Design review of the part built by this model. Coordinates are the model's own, in mm. Face numbers are marked on the shaded views. A direction names the side the tool comes from. Coordinates: 2 decimals unless noted, no trailing zeros. Loops run counter-clockwise (first coordinate to the right, second up) from the corner with the lowest first, then second, coordinate; pieces in that order, holes last. Notation, with made-up numbers: (-39.5, 29) -> (8.5, 29) arc R14 cw to (8.5, 35) -> close; hole circle Ø7 at (71, 21). An arc over 180 degrees is marked (long way). Answer in a Markdown table with one row per item.
```python
from build123d import *

# Parameters (mm, degrees)
SKETCH_1_R      = 9.9
SKETCH_1_R_2    = 1.85
EXTRUDE_1_DEPTH = 7
SKETCH_2_R      = 12.5
SKETCH_2_R_2    = 1.85
EXTRUDE_2_DEPTH = 2.5
SKETCH_3_R      = 3.75
EXTRUDE_3_DEPTH = 6.3
CHAMFER_1_SIZE  = 2


with BuildPart() as part:
    # 草图1 → 凸台-拉伸1 (new body)
    with BuildSketch(Plane(origin=(0, 0, 0), x_dir=(1, 0, 0), z_dir=(0, 1, 0))):
        with Locations(Location((0, 0, 0), (0, 0, 270))):
            Circle(SKETCH_1_R)
        with Locations(Location((6, 0, 0), (0, 0, 270))):
            Circle(SKETCH_1_R_2, mode=Mode.SUBTRACT)
        with Locations(Location((0, -6, 0), (0, 0, 270))):
            Circle(SKETCH_1_R_2, mode=Mode.SUBTRACT)
        with Locations(Location((-6, 0, 0), (0, 0, 270))):
            Circle(SKETCH_1_R_2, mode=Mode.SUBTRACT)
        with Locations(Location((0, 6, 0), (0, 0, 270))):
            Circle(SKETCH_1_R_2, mode=Mode.SUBTRACT)
    extrude(amount=EXTRUDE_1_DEPTH)

    # 草图2 → 凸台-拉伸2 (add)
    with BuildSketch(Plane(origin=(0, 7, 0), x_dir=(1, 0, 0), z_dir=(0, 1, 0))):
        with Locations(Location((0, 0, 0), (0, 0, 270))):
            Circle(SKETCH_2_R)
        with Locations(Location((-6, 0, 0), (0, 0, 270))):
            Circle(SKETCH_2_R_2, mode=Mode.SUBTRACT)
        with Locations(Location((0, -6, 0), (0, 0, 270))):
            Circle(SKETCH_2_R_2, mode=Mode.SUBTRACT)
        with Locations(Location((6, 0, 0), (0, 0, 270))):
            Circle(SKETCH_2_R_2, mode=Mode.SUBTRACT)
        with Locations(Location((0, 6, 0), (0, 0, 270))):
            Circle(SKETCH_2_R_2, mode=Mode.SUBTRACT)
    extrude(amount=EXTRUDE_2_DEPTH)

    # 草图3 → 凸台-拉伸3 (add)
    # profile 1 of 8: a face of its own
    with BuildSketch(Plane(origin=(0, 9.5, 0), x_dir=(1, 0, 0), z_dir=(0, 1, 0))):
        with BuildLine():
            Line((2.25, 0), (-2.25, 0))
            ThreePointArc((-2.25, 0), (-6, -3.75), (-9.75, 0))
            Line((-9.75, 0), (-12.5, 0))
            ThreePointArc((-12.5, 0), (-3.952847075, -11.858541226), (10, -7.5))
            ThreePointArc((10, -7.5), (11.858541226, -3.952847075), (12.5, 0))
            Line((12.5, 0), (9.75, 0))
            ThreePointArc((9.75, 0), (6, -3.75), (2.25, 0))
        make_face()
        with Locations(Location((0, -6, 0), (0, 0, 270))):
            Circle(SKETCH_3_R, mode=Mode.SUBTRACT)
    # profile 2 of 8: a face of its own
    with BuildSketch(Plane(origin=(0, 9.5, 0), x_dir=(1, 0, 0), z_dir=(0, 1, 0))):
        with BuildLine():
            ThreePointArc((-9.75, 0), (-6, 3.75), (-2.25, 0))
            Line((-2.25, 0), (2.25, 0))
            ThreePointArc((2.25, 0), (6, 3.75), (9.75, 0))
            Line((9.75, 0), (12.5, 0))
            ThreePointArc((12.5, 0), (11.858541226, 3.952847075), (10, 7.5))
            ThreePointArc((10, 7.5), (-3.952847075, 11.858541226), (-12.5, 0))
            Line((-12.5, 0), (-9.75, 0))
        make_face()
        with Locations(Location((0, 6, 0), (0, 0, 270))):
            Circle(SKETCH_3_R, mode=Mode.SUBTRACT)
    # profile 3 of 8: a face of its own
    with BuildSketch(Plane(origin=(0, 9.5, 0), x_dir=(1, 0, 0), z_dir=(0, 1, 0))):
        with BuildLine():
            ThreePointArc((10, 7.5), (11.858541226, 3.952847075), (12.5, 0))
            Line((12.5, 0), (25.5, 0))
            ThreePointArc((25.5, 0), (27.696699141, 5.303300859), (33, 7.5))
            Line((33, 7.5), (10, 7.5))
        make_face()
    # profile 4 of 8: a face of its own
    with BuildSketch(Plane(origin=(0, 9.5, 0), x_dir=(1, 0, 0), z_dir=(0, 1, 0))):
        with BuildLine():
            Line((25.5, 0), (12.5, 0))
            ThreePointArc((12.5, 0), (11.858541226, -3.952847075), (10, -7.5))
            Line((10, -7.5), (33, -7.5))
            ThreePointArc((33, -7.5), (27.696699141, -5.303300859), (25.5, 0))
        make_face()
    # profile 5 of 8: a face of its own
    with BuildSketch(Plane(origin=(0, 9.5, 0), x_dir=(1, 0, 0), z_dir=(0, 1, 0))):
        with BuildLine():
            ThreePointArc((33, 7.5), (27.696699141, 5.303300859), (25.5, 0))
            Line((25.5, 0), (28.65, 0))
            ThreePointArc((28.65, 0), (33, 4.35), (37.35, 0))
            Line((37.35, 0), (40.5, 0))
            ThreePointArc((40.5, 0), (38.303300859, 5.303300859), (33, 7.5))
        make_face()
    # profile 6 of 8: a face of its own
    with BuildSketch(Plane(origin=(0, 9.5, 0), x_dir=(1, 0, 0), z_dir=(0, 1, 0))):
        with BuildLine():
            Line((28.65, 0), (25.5, 0))
            ThreePointArc((25.5, 0), (27.696699141, -5.303300859), (33, -7.5))
            ThreePointArc((33, -7.5), (38.303300859, -5.303300859), (40.5, 0))
            Line((40.5, 0), (37.35, 0))
            ThreePointArc((37.35, 0), (33, -4.35), (28.65, 0))
        make_face()
    # profile 7 of 8: a face of its own
    with BuildSketch(Plane(origin=(0, 9.5, 0), x_dir=(1, 0, 0), z_dir=(0, 1, 0))):
        with BuildLine():
            ThreePointArc((33, 7.5), (27.696699141, 5.303300859), (25.5, 0))
            Line((25.5, 0), (28.65, 0))
            ThreePointArc((28.65, 0), (33, 4.35), (37.35, 0))
            Line((37.35, 0), (40.5, 0))
            ThreePointArc((40.5, 0), (38.303300859, 5.303300859), (33, 7.5))
        make_face()
    # profile 8 of 8: a face of its own
    with BuildSketch(Plane(origin=(0, 9.5, 0), x_dir=(1, 0, 0), z_dir=(0, 1, 0))):
        with BuildLine():
            Line((28.65, 0), (25.5, 0))
            ThreePointArc((25.5, 0), (27.696699141, -5.303300859), (33, -7.5))
            ThreePointArc((33, -7.5), (38.303300859, -5.303300859), (40.5, 0))
            Line((40.5, 0), (37.35, 0))
            ThreePointArc((37.35, 0), (33, -4.35), (28.65, 0))
        make_face()
    extrude(amount=EXTRUDE_3_DEPTH)

    # 倒角1
    # the kernel refuses this chamfer: 2 mm, written as the material it adds along each edge
    with BuildSketch(Plane(origin=(0, 9.5, 6), x_dir=(0, 0, 1), z_dir=(-1, 0, 0))) as chamfer_1_piece_1_section:
        Polygon((3.75 - CHAMFER_1_SIZE, 0), (3.75, CHAMFER_1_SIZE), (3.75, 0), align=None)
    chamfer_1_piece_1 = revolve(axis=Axis((0, 9.5, 6), (0, 1, 0)), mode=Mode.PRIVATE)
    chamfer_1_piece_1 = chamfer_1_piece_1 - Plane(origin=(0, 10.553600351, 6), x_dir=(0, 0, 1), z_dir=(0, -1, 0)) * Cylinder(1.85, 15, mode=Mode.PRIVATE)
    add(chamfer_1_piece_1)
    with BuildSketch(Plane(origin=(-6, 9.5, 0), x_dir=(-1, 0, 0), z_dir=(0, 0, 1))) as chamfer_1_piece_2_section:
        Polygon((3.75 - CHAMFER_1_SIZE, 0), (3.75, -CHAMFER_1_SIZE), (3.75, 0), align=None)
    chamfer_1_piece_2 = revolve(axis=Axis((-6, 9.5, 0), (0, -1, 0)), mode=Mode.PRIVATE)
    chamfer_1_piece_2 = chamfer_1_piece_2 - Plane(origin=(-6, 10.553600351, 0), x_dir=(0, 0, 1), z_dir=(0, -1, 0)) * Cylinder(1.85, 15, mode=Mode.PRIVATE)
    add(chamfer_1_piece_2)
    with BuildSketch(Plane(origin=(0, 9.5, -6), x_dir=(0, 0, 1), z_dir=(-1, 0, 0))) as chamfer_1_piece_3_section:
        Polygon((3.75 - CHAMFER_1_SIZE, 0), (3.75, CHAMFER_1_SIZE), (3.75, 0), align=None)
    chamfer_1_piece_3 = revolve(axis=Axis((0, 9.5, -6), (0, 1, 0)), mode=Mode.PRIVATE)
    chamfer_1_piece_3 = chamfer_1_piece_3 - Plane(origin=(0, 10.553600351, -6), x_dir=(0, 0, 1), z_dir=(0, -1, 0)) * Cylinder(1.85, 16, mode=Mode.PRIVATE)
    add(chamfer_1_piece_3)
    with BuildSketch(Plane(origin=(6, 9.5, 0), x_dir=(1, 0, 0), z_dir=(0, 0, -1))) as chamfer_1_piece_4_section:
        Polygon((3.75 - CHAMFER_1_SIZE, 0), (3.75, -CHAMFER_1_SIZE), (3.75, 0), align=None)
    chamfer_1_piece_4 = revolve(axis=Axis((6, 9.5, 0), (0, -1, 0)), mode=Mode.PRIVATE)
    chamfer_1_piece_4 = chamfer_1_piece_4 - Plane(origin=(6, 10.553600351, 0), x_dir=(0, 0, 1), z_dir=(0, -1, 0)) * Cylinder(1.85, 15, mode=Mode.PRIVATE)
    add(chamfer_1_piece_4)


solid = part.part
```
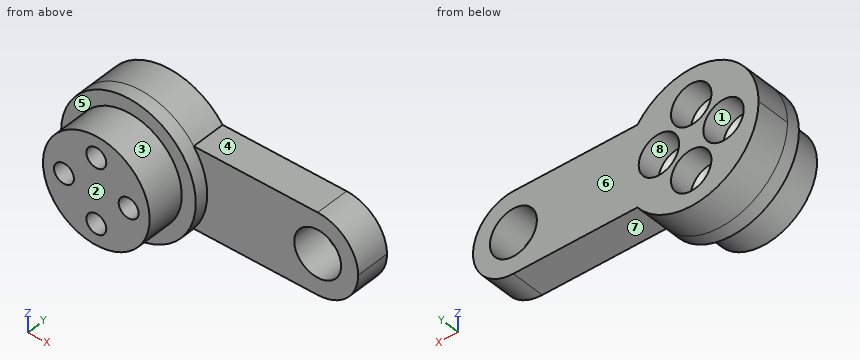
(1) Take a section at C-C on z = 6. Give the boundary of the cut face in (x, y), and give its area (3 significant figures).
Evaluation:
| item | result |
|---|---|
| outline | (-10.97, 7) -> (-7.87, 7) -> (-7.87, 0) -> (-1.85, 0) -> (-1.85, 9.6) -> (-3.75, 11.5) -> (-3.75, 15.8) -> (-10.97, 15.8) -> close; (1.85, 0) -> (7.87, 0) -> (7.87, 7) -> (10.97, 7) -> (10.97, 9.5) -> (37.5, 9.5) -> (37.5, 15.8) -> (3.75, 15.8) -> (3.75, 11.5) -> (1.85, 9.6) -> close |
| area | 392 mm² |
(2) Take a section at A-A on x = 0. Give the boundary of the cut face in (y, z).
Evaluation:
| item | result |
|---|---|
| outline | (0, -9.9) -> (7, -9.9) -> (7, -12.5) -> (15.8, -12.5) -> (15.8, -9.75) -> (11.5, -9.75) -> (9.6, -7.85) -> (0, -7.85) -> close; (0, -4.15) -> (9.6, -4.15) -> (11.5, -2.25) -> (15.8, -2.25) -> (15.8, 2.25) -> (11.5, 2.25) -> (9.6, 4.15) -> (0, 4.15) -> close; (0, 7.85) -> (9.6, 7.85) -> (11.5, 9.75) -> (15.8, 9.75) -> (15.8, 12.5) -> (7, 12.5) -> (7, 9.9) -> (0, 9.9) -> close |
(3) For pin 1 (4.5 mm diameter, centred on x = 0, z = 6, fed in from -Y); pin 2 (5 mm diameter, centred on x = 7, y = 6.5, fed in from -Z); pin 3 (2 mm diameter, centred on y = 8, z = -2.5, fed in from +X); pin 4 (12 mm diameter, centred on x = 21.5, z = 3, fed in from -Y), all flat-tipped, find the tip position at first contact; note any pin that passes through.
Evaluation:
| item | result |
|---|---|
| pin 1 | stops at y = 0 |
| pin 2 | stops at z = -11.64 |
| pin 3 | stops at x = 12.41 |
| pin 4 | stops at y = 9.5 |
(4) Tool access review of the marked faces 4, 5, 6, 7 and 8: name each direction out of +Z, -Z, +X, -X, +Y, -Y from which nothing blocks a thin tool from reaching the whole face with its end or side.
Evaluation:
| item | result |
|---|---|
| face 4 | +Z, +X, +Y, -Y |
| face 5 | -Y |
| face 6 | +Z, -Z, +X, -X, +Y |
| face 7 | -Z, +X, +Y, -Y |
| face 8 | +Y |
(5) Draft analysis for pull direction Z (two halves, no side actions). For the marked faces 1, 2 and 3, state which applies: pulls with the +Z half, pulls with the -Z half, needs draft (parallel to the pull), parting line crosses it, or undercut.
Evaluation:
| item | result |
|---|---|
| face 1 | undercut |
| face 2 | needs draft |
| face 3 | parting line crosses it |
(6) Take a section at D-D on y = 3.25. Give the boundary of the cut face in (x, z), and give its area (3 significant figures).
Evaluation:
| item | result |
|---|---|
| outline | circle Ø19.8 at (0, 0); hole circle Ø3.7 at (-6, 0); hole circle Ø3.7 at (0, -6); hole circle Ø3.7 at (0, 6); hole circle Ø3.7 at (6, 0) |
| area | 265 mm² |
(7) To check wall thickness, follow probe 1 along Y at (x, z) = (18, -4.75); probe 2 along Z at (x, y) = (-6, 13.8); probe 3 along X at (y, z) = (9, 7). State the ranges of each line that lie inside material, in increasing order.
Evaluation:
| item | result |
|---|---|
| probe 1 | y = 9.5 to 15.8 |
| probe 2 | z = -10.97 to -3.75, 3.75 to 10.97 |
| probe 3 | x = -10.36 to -1.56, 1.56 to 10.36 |
(8) Take a section at B-B on y = 14.25. Give the boundary of the cut face in (x, z), and give its area (3 significant figures).
Evaluation:
| item | result |
|---|---|
| outline | (10, -7.5) -> (33, -7.5) arc R7.5 ccw to (33, 7.5) -> (10, 7.5) arc R12.5 ccw (long way) to start; hole circle Ø7.5 at (-6, 0); hole circle Ø7.5 at (0, -6); hole circle Ø7.5 at (0, 6); hole circle Ø7.5 at (6, 0); hole circle Ø8.7 at (33, 0) |
| area | 663 mm² |
